from build123d import *

# Parameters (mm, degrees)
SKETCH1_R           = 1.5625
BOSS_EXTRUDE1_DEPTH = 3
BOSS_EXTRUDE2_DEPTH = 13
CUT_EXTRUDE1_DEPTH  = 11.5
SKETCH4_R           = 1.96
CUT_EXTRUDE2_DEPTH  = 7
CHAMFER1_SIZE       = 1
FILLET1_R           = 6
CHAMFER2_SIZE       = 3.4
CHAMFER3_SIZE       = 0.5
SKETCH5_R           = 2.8
CUT_EXTRUDE3_DEPTH  = 1
SKETCH6_R           = 1.25
SKETCH6_R_2         = 2
BOSS_EXTRUDE3_DEPTH = 1
CHAMFER4_SIZE       = 0.25


with BuildPart() as part:
    # Sketch1 → Boss-Extrude1 (new body)
    with BuildSketch(Plane(origin=(0, 0, 0), x_dir=(1, 0, 0), z_dir=(0, 1, 0))):
        with BuildLine():
            Line((3.181980515, -15.181980515), (18.5, 0.136038969))
            Line((18.5, 0.136038969), (18.5, 8))
            ThreePointArc((18.5, 8), (17.181980515, 11.181980515), (14, 12.5))
            Line((14, 12.5), (6, 12.5))
            Line((6, 12.5), (1, 7.5))
            Line((1, 7.5), (-4.5, 2))
            Line((-4.5, 2), (-4.5, -6.5))
            Line((-4.5, -6.5), (-4.5, -12))
            ThreePointArc((-4.5, -12), (-1.722075446, -16.157457896), (3.181980515, -15.181980515))
        make_face()
        with Locations((0, -12)):
            Circle(SKETCH1_R, mode=Mode.SUBTRACT)
        with Locations((14, 8)):
            Circle(SKETCH1_R, mode=Mode.SUBTRACT)
    extrude(amount=BOSS_EXTRUDE1_DEPTH)

    # Sketch2 → Boss-Extrude2 (add)
    with BuildSketch(Plane.ZY.offset(4.5)):
        with BuildLine():
            Line((-8, 0), (8, 0))
            Line((8, 0), (8, 3))
            ThreePointArc((8, 3), (7.199378454, 4.60097271), (6.08276253, 6))
            Line((6.08276253, 6), (-6.08276253, 6))
            ThreePointArc((-6.08276253, 6), (-7.199378454, 4.60097271), (-8, 3))
            Line((-8, 3), (-8, 0))
        make_face()
    extrude(amount=-BOSS_EXTRUDE2_DEPTH)

    # Sketch3 → Cut-Extrude1 (cut)
    with BuildSketch(Plane.ZY.offset(4.5)):
        with BuildLine():
            Line((-6.75, 0), (6.75, 0))
            ThreePointArc((6.75, 0), (6.516244021, 1.760983776), (5.831166264, 3.4))
            Line((5.831166264, 3.4), (-5.831166264, 3.4))
            ThreePointArc((-5.831166264, 3.4), (-6.516244021, 1.760983776), (-6.75, 0))
        make_face()
    extrude(amount=-CUT_EXTRUDE1_DEPTH, mode=Mode.SUBTRACT)

    # Sketch4 → Cut-Extrude2 (cut, through all)
    with BuildSketch(Plane(origin=(0, 6, 0), x_dir=(1, 0, 0), z_dir=(0, 1, 0))):
        Circle(SKETCH4_R)
    extrude(amount=-CUT_EXTRUDE2_DEPTH, mode=Mode.SUBTRACT)

    # Chamfer1
    chamfer1_edges = [part.edges().sort_by_distance(p)[0] for p in [
        (8.5, 3, 0),
    ]]
    chamfer(chamfer1_edges, length=CHAMFER1_SIZE)

    # Fillet1
    fillet1_edges = [part.edges().sort_by_distance(p)[0] for p in [
        (18.5, 1.5, -0.136038969),
    ]]
    fillet(fillet1_edges, radius=FILLET1_R)

    # Chamfer2
    chamfer2_edges = [part.edges().sort_by_distance(p)[0] for p in [
        (-4.5, 0, -7.375),
    ]]
    chamfer(chamfer2_edges, length=CHAMFER2_SIZE)

    # Chamfer3
    chamfer3_edges = [part.edges().sort_by_distance(p)[0] for p in [
        (7, 1.760983776, -6.516244021),
        (7, 3.4, 0),
        (7, 1.760983776, 6.516244021),
    ]]
    chamfer(chamfer3_edges, length=CHAMFER3_SIZE)

    # Sketch5 → Cut-Extrude3 (cut)
    with BuildSketch(Plane(origin=(0, 3, 0), x_dir=(1, 0, 0), z_dir=(0, 1, 0))):
        with Locations((0, -12)):
            Circle(SKETCH5_R)
        with Locations((14, 8)):
            Circle(SKETCH5_R)
    extrude(amount=-CUT_EXTRUDE3_DEPTH, mode=Mode.SUBTRACT)

    # Sketch6 → Boss-Extrude3 (add)
    with BuildSketch(Plane.XZ):
        with Locations((4.5, 9.75)):
            Circle(SKETCH6_R)
        with Locations((11.5, 0)):
            Circle(SKETCH6_R_2)
        with Locations((7.5, -9.5)):
            Circle(SKETCH6_R)
    extrude(amount=BOSS_EXTRUDE3_DEPTH)

    # Chamfer4
    chamfer4_edges = [part.edges().sort_by_distance(p)[0] for p in [
        (-1.722075446, 3, 16.157457896),
        (3.25, -1, 9.75),
        (9.5, -1, 0),
        (6.25, -1, -9.5),
        (9.962310601, 3, 8.401650429),
        (17.181980515, 3, -11.181980515),
        (10, 3, -12.5),
        (-4.5, 3, 10),
        (3.75, 3, -10.25),
        (8.5, 6, 0),
        (18.5, 3, -5.310660172),
        (18.043277195, 3, -0.325219749),
    ]]
    chamfer(chamfer4_edges, length=CHAMFER4_SIZE)


solid = part.part
Input: part model. Units: mm. Frame: model coordinates. A direction names the side the tool comes from. Round coordinates to 2 decimals unless told otherwise and drop trailing zeros. Order: outer loops, then holes, each group sorted by start corner. A loop starts at its lowest first (then second) coordinate and runs counter-clockwise, first axis right, second up. Notation, with made-up numbers: (62, 59.25) - (85, 59.25) arc R23 cw to (85, 95.25) - close; hole circle Ø5 at (56.5, 68). An arc over 180 degrees is marked (long way). Answer as a JSON object with one key per item and string values. Group by question number.
(1) Material intervals for probe 1 along X at (y, z) = (4.45, 0); probe 2 along Z at (x, y) = (0, 0.75); probe 3 along Z at (x, y) = (0, 2.4), sorted ascending. Write a range as from..to.
(2) Pin query (flat end, axial travel): P1, Ø5, axis at x = 14, z = -8, coming from the -Y side; P2, Ø3.5, axis at x = 0, y = 1.5, coming from the -Z side; P3, Ø0.9, axis at y = 5, z = 3.5, coming from the +X side. Return the tip coordinate at first contact, or that it passes through.
(3) Cut plane C-C (x = 4.5). Return loops of the section in (y, z), then the cut area to 3 significant figures.
(4) Cut plane B-B (z = -3.75). Return loops of the section in (x, y), then the cut area to 3 significant figures.
(5) Cut plane A-A (x = 0). Return loops of the section in (y, z).
(6) Cut plane D-D (z = 9.75). Return loops of the section in (x, y).
(7) Draft query along X for faces 6 (the face through (0, 2, 14)), 7 (the face through (9, 3.5, -0.1)), 8 (the face through (10, 1, -12.5)), 9 (the face through (-0.2, 0.99, 10.45)). Return one class per face: released by +X, released by -X, zero draft, split by the parting line, or undercut.
(8) Reachability of faces 1 (the face through (-3.2, 2.1, -7.1)), 2 (the face through (11.778, 2.507, -6.296)), 3 (the face through (7, 1, 0)), 4 (the face through (6.25, -0.37, -9.45)), 5 (the face through (10, 3, 2)) from +Z, -Z, +X, -X, +Y, -Y: full face, straight path, thin tool, end or side. Return the list, or none.
Here are the results:
{
 "1": {"probe 1": "x = -4.5..-1.96, 1.96..8.5", "probe 2": "z = -8..-6.71, 6.71..10.44, 13.56..16.5", "probe 3": "z = -8..-6.31, 6.31..9.2, 14.8..16.5"},
 "2": {"P1": "stops at y = 0", "P2": "stops at z = -8.25", "P3": "stops at x = 8.5"},
 "3": {"outline": "(-1, 8.75) - (-0.75, 8.5) - (0, 8.5) - (0, 6.75) arc R6.75 cw to (3.4, 5.83) - (3.4, -5.83) arc R6.75 cw to (0, -6.75) - (0, -11) - (2.75, -11) - (3, -10.65) - (3, -8) arc R8.54 ccw to (6, -6.08) - (6, 6.08) arc R8.54 ccw to (3, 8) - (3, 13.51) - (2.75, 13.86) - (0, 13.86) - (0, 11) - (-0.75, 11) - (-1, 10.75) - close", "area": "76.2 mm^2"},
 "4": {"outline": "(-4.5, 3.4) - (6.5, 3.4) - (7, 2.9) - (7, 0) - (18.5, 0) - (18.5, 2.75) - (18.25, 3) - (9.5, 3) - (8.5, 4) - (8.5, 5.75) - (8.25, 6) - (-4.5, 6) - close", "area": "69.5 mm^2"},
 "5": {"outline": "(0, -8) - (3, -8) arc R8.54 ccw to (6, -6.08) - (6, -1.96) - (3.4, -1.96) - (3.4, -5.83) arc R6.75 cw to (0, -6.75) - close; (0, 6.75) arc R6.75 cw to (3.4, 5.83) - (3.4, 1.96) - (6, 1.96) - (6, 6.08) arc R8.54 ccw to (3, 8) - (3, 9.2) - (2, 9.2) - (2, 10.44) - (0, 10.44) - close; (0, 13.56) - (2, 13.56) - (2, 14.8) - (3, 14.8) - (3, 16.25) - (2.75, 16.5) - (0, 16.5) - close"},
 "6": {"outline": "(-4.5, 0) - (3.25, 0) - (3.25, -0.75) - (3.5, -1) - (5.5, -1) - (5.75, -0.75) - (5.75, 0) - (8.61, 0) - (8.61, 2.75) - (8.26, 3) - (1.67, 3) - (1.67, 2) - (-1.67, 2) - (-1.67, 3) - (-4.25, 3) - (-4.5, 2.75) - close"},
 "7": {"face 6": "undercut", "face 7": "released by +X", "face 8": "zero draft", "face 9": "undercut"},
 "8": {"face 1": "-Z, -X, -Y", "face 2": "+Y", "face 3": "-X, -Y", "face 4": "-Y", "face 5": "+X, +Y"}
}
